Could you check a few things on this drawing? It's one solid part, dimensions in mm from its lowest x, y, z. Coordinates: 2 decimals unless noted, no trailing zeros. Loops run counter-clockwise (first coordinate to the right, second up) from the corner with the lowest first, then second, coordinate; pieces in that order, holes last.
1) If I drill on line 1 along X through (y, z) = (58, 0.4) (1 decimal); line 2 along Y through (x, z) = (61, 2.55), over which ranges is the centre line in solid material (lowest first)?
2) Imagine slicing it at B-B on x = 54.5. Please give me the cut outline in (y, z) (1 decimal), plus the area to 3 significant figures.
3) Will these pins go through, and if not, where does the flat tip stop? P1, Ø1, axis at x = 29.5, y = 23.5, coming from the -Z side; P2, Ø1.4, axis at y = 8, z = 2, coming from the +X side; P3, Ø0.9, axis at y = 2, z = 0.5, coming from the -X side; P4, Ø1.4, axis at x = 62.5, z = 1.5, coming from the -Y side.
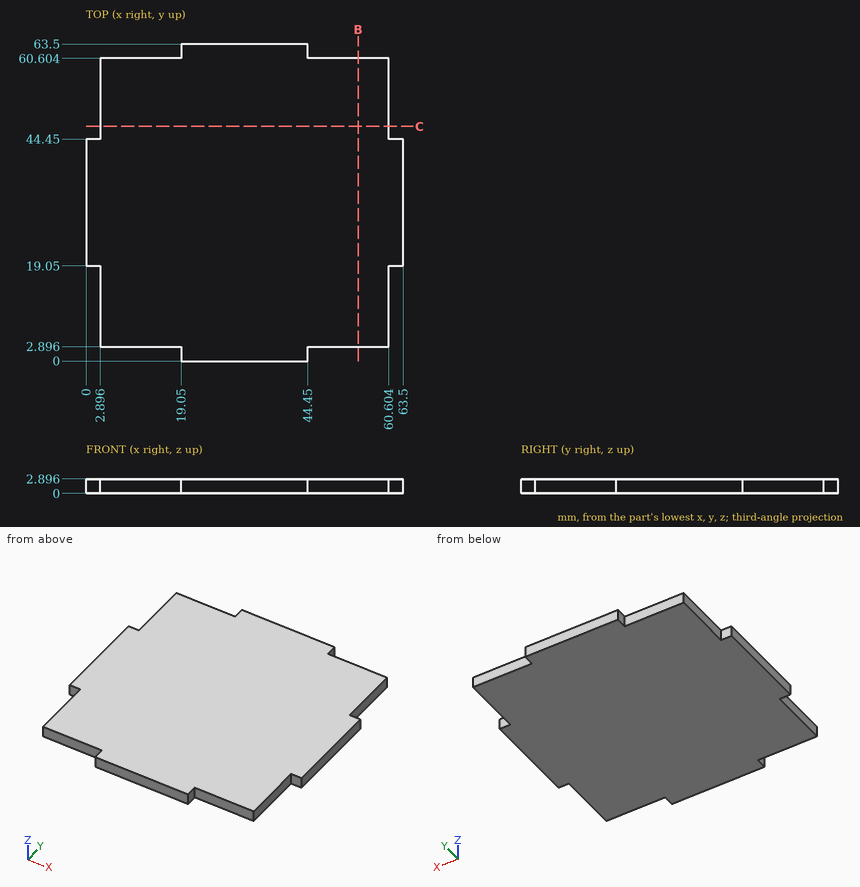
Filled in:
1. line 1: x = 2.9 to 60.6
1. line 2: y = 19.05 to 44.45
2. outline: (2.9, 0) - (60.6, 0) - (60.6, 2.9) - (2.9, 2.9) - close
2. area: 167 mm2
3. P1: stops at z = 0
3. P2: stops at x = 60.6
3. P3: stops at x = 19.05
3. P4: stops at y = 19.05
